Here's the drawing with two shaded views (mm, measured from the low corner). I have some questions. A direction names the side the tool comes from. Give positions to 0.01 mm unless a question says otherwise; leave off trailing zeros. Write each loop counter-clockwise with the first axis right and the second up, starting at its lowest first coordinate (ties: lowest second). Pieces come first, ordered by that corner, then holes.
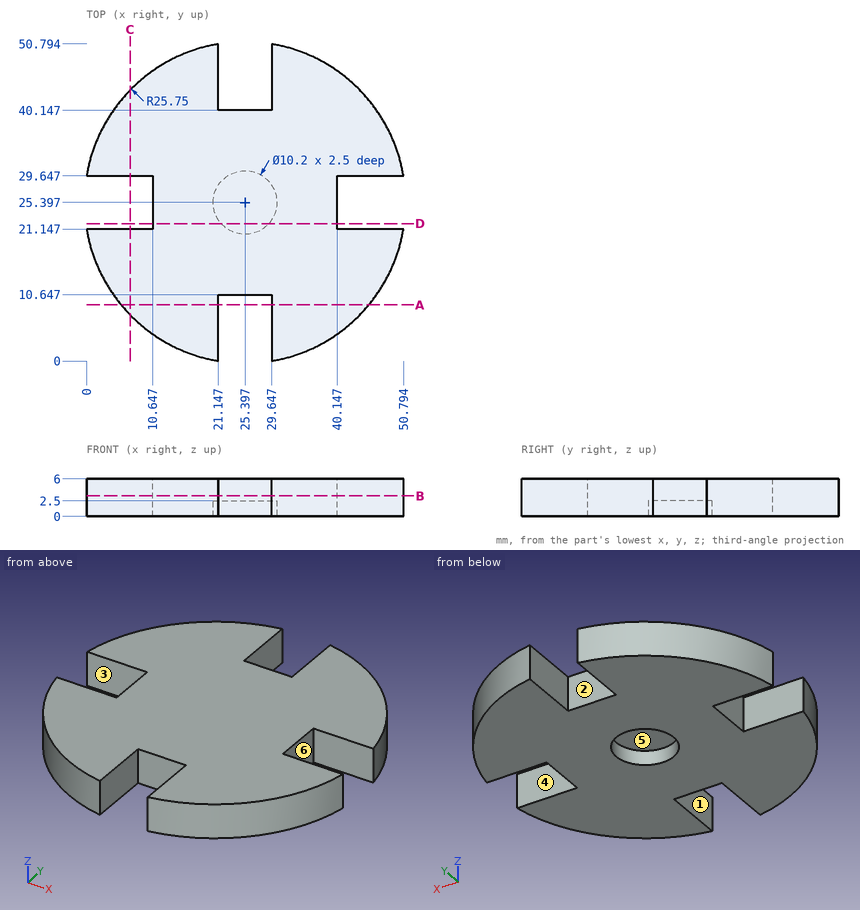
1) Please list where these lines run through material, in increasing order: L1, parallel to Y at x = 42.5, z = 1.25 (1 decimal); L2, parallel to X at y = 26.5, z = 2.9; L3, parallel to X at y = 8, z = 1.
Values follow:
L1: y = 6.1 to 21.1, 29.6 to 44.6
L2: x = 10.65 to 40.15
L3: x = 6.41 to 21.15, 29.65 to 44.38
2) Suppose I cut it at B-B on z = 3.3. Write out the boundary of the cut face in (x, y).
Values follow:
outline: (0, 21.15) arc R25.75 ccw to (21.15, 0) - (21.15, 10.65) - (29.65, 10.65) - (29.65, 0) arc R25.75 ccw to (50.79, 21.15) - (40.15, 21.15) - (40.15, 29.65) - (50.79, 29.65) arc R25.75 ccw to (29.65, 50.79) - (29.65, 40.15) - (21.15, 40.15) - (21.15, 50.79) arc R25.75 ccw to (0, 29.65) - (10.65, 29.65) - (10.65, 21.15) - close
3) For the marked faces 1, 2 and 3, which set-ups out of +Z, -Z, +X, -X, +Y, -Y let a thin tool reach every point of the face, with its end or its side?
Values follow:
face 1: +Z, -Z, -Y
face 2: +Z, -Z, +Y
face 3: +Z, -Z, -X
4) Suppose I cut it at A-A on y = 9. Write out the boundary of the cut face in (x, z), plus the area to 3 significant figures.
Values follow:
outline: (5.54, 0) - (21.15, 0) - (21.15, 6) - (5.54, 6) - close; (29.65, 0) - (45.25, 0) - (45.25, 6) - (29.65, 6) - close
area: 187 mm2
5) Suppose I cut it at D-D on y = 22. Write out the boundary of the cut face in (x, z), plus the area to 3 significant figures.
Values follow:
outline: (10.65, 0) - (21.59, 0) - (21.59, 2.5) - (29.2, 2.5) - (29.2, 0) - (40.15, 0) - (40.15, 6) - (10.65, 6) - close
area: 158 mm2
6) Suppose I cut it at C-C on x = 7. Write out the boundary of the cut face in (y, z), plus the area to 3 significant figures.
Values follow:
outline: (7.38, 0) - (21.15, 0) - (21.15, 6) - (7.38, 6) - close; (29.65, 0) - (43.41, 0) - (43.41, 6) - (29.65, 6) - close
area: 165 mm2
7) If we mould it in two halves opening along X, with no side actions, what happens to the marked faces 4, 5 and 6? For each: +X half, -X half, draft (parallel to the pull), parting line (faces both ways), or undercut.
Values follow:
face 4: draft
face 5: undercut
face 6: +X half
8) For pin 1 Ø1.8 at (x, z) = (46.5, 4) entering from -Y; pin 2 Ø3 at (x, z) = (23.5, 2) entering from -Y; pin 3 Ø2 at (y, z) = (27.5, 1.5) entering from +X, each with a flat end and sliding along its axis, tell me the tip position at first contact or that it passes through.
Values follow:
pin 1: stops at y = 9.43
pin 2: stops at y = 10.65
pin 3: stops at x = 40.15
